from build123d import *

# Parameters (mm, degrees)
SKETCH1_R           = 2.25
BOSS_EXTRUDE1_DEPTH = 15
SKETCH2_R           = 2.25
CUT_EXTRUDE1_DEPTH  = 20
FILLET1_R           = 10


with BuildPart() as part:
    # Sketch1 → Boss-Extrude1 (new body)
    with BuildSketch(Plane(origin=(0, 0, 0), x_dir=(1, 0, 0), z_dir=(0, 1, 0))):
        with BuildLine():
            Line((-87.85411681, -7.5), (-62.85411681, -7.5))
            ThreePointArc((-62.85411681, -7.5), (1.256140371, -63.287535197), (63.102218661, -5))
            Line((63.102218661, -5), (73.102218661, -5))
            Line((73.102218661, -5), (73.102218661, -1))
            Line((73.102218661, -1), (55.290957669, -1))
            ThreePointArc((55.290957669, -1), (-55.3, 0), (55.290957669, 1))
            Line((55.290957669, 1), (73.102218661, 1))
            Line((73.102218661, 1), (73.102218661, 5))
            Line((73.102218661, 5), (63.102218661, 5))
            ThreePointArc((63.102218661, 5), (1.256140371, 63.287535197), (-62.85411681, 7.5))
            Line((-62.85411681, 7.5), (-87.85411681, 7.5))
            Line((-87.85411681, 7.5), (-87.85411681, -7.5))
        make_face()
        with Locations(Location((-80.85411681, 0, 0), (0, 0, 270))):
            Circle(SKETCH1_R, mode=Mode.SUBTRACT)
        with Locations(Location((-65.85411681, 0, 0), (0, 0, 270))):
            Circle(SKETCH1_R, mode=Mode.SUBTRACT)
    extrude(amount=BOSS_EXTRUDE1_DEPTH)

    # Sketch2 → Cut-Extrude1 (cut)
    with BuildSketch(Plane.XY.offset(5)):
        with Locations((68.102218661, 7.5)):
            Circle(SKETCH2_R)
    extrude(amount=-CUT_EXTRUDE1_DEPTH, mode=Mode.SUBTRACT)

    # Fillet1
    fillet1_edges = [part.edges().sort_by_distance(p)[0] for p in [
        (-62.85411681, 7.5, 7.5),
        (-62.85411681, 7.5, -7.5),
    ]]
    fillet(fillet1_edges, radius=FILLET1_R)


solid = part.part
CAD build for the part. Positions are in the model's coordinates, mm. A direction names the side the tool comes from. Give positions to 0.01 mm unless a question says otherwise; leave off trailing zeros. Loops run counter-clockwise (first coordinate to the right, second up) from the corner with the lowest first, then second, coordinate; pieces in that order, holes last. Notation, with made-up numbers: M 35,30.25 L 77,30.25 A25 ccw 77,65.25 Z; hole C -2,-9.5 d1. An arc over 180 degrees is marked long. Answer in a Markdown table with one row per item. Add a question column.
Item 1: Band-saw the part on C-C on z = 17.5. Give the cut face in (x, y), then the cut area to 3 significant figures.
Item 2: Tool access for faces 5 (the face through (64, 7, 1)), 6 (the face through (66, 9, 5)), 7 (the face through (-79, 7, -7.5)): list every direction of +Z, -Z, +X, -X, +Y, -Y with a clear straight run to the whole face (end or side of a thin tool).
Item 3: Drop flat-ended pins along their axis: P1, Ø10, axis at x = -23.5, z = -42.5, coming from the -Y side; P2, Ø1, axis at y = 6, z = 40.5, coming from the +X side; P3, Ø3, axis at x = 67.5, y = 8.5, coming from the -Z side; P4, Ø5, axis at x = 66.5, y = 9, coming from the +Z side. Give the stop position or say it passes through.
Item 4: Band-saw the part on A-A on x = 0. Give the cut face in (y, z).
Item 5: Probe probe 1 along X at (y, z) = (8.75, 0); probe 2 along Z at (x, y) = (1, 8.25); probe 3 along Z at (x, y) = (65, 10.5). List the from-to ranges inside material, lowest first.
Item 6: Mould opens along Y. For faces 1 (the face through (70, 9, -5)), 2 (the face through (-55.4, 0, -5)), 3 (the face through (65.854, 7.599, 3.028)), 4 (the face through (65.854, 7.599, -2.972)) say: +Y half, -Y half, draft (parallel to the pull), parting line (faces both ways), or undercut.
Item 7: Band-saw the part on D-D on x = -73. Give the cut face in (y, z).
Item 8: Band-saw the part on B-B on y = 7.5. Give the cut face in (x, z).
Reply:
| question | item | result |
|---|---|---|
| 1 | outline | M -60.83,0 L -52.46,0 L -52.46,15 L -60.83,15 Z; M 52.46,0 L 60.83,0 L 60.83,15 L 52.46,15 Z |
| 1 | area | 251 mm^2 |
| 2 | face 5 | +X, +Y, -Y |
| 2 | face 6 | +Z, +X, +Y, -Y |
| 2 | face 7 | -Z, -X, +Y, -Y |
| 3 | P1 | passes through |
| 3 | P2 | stops at x = 49.06 |
| 3 | P3 | stops at z = -5 |
| 3 | P4 | stops at z = 5 |
| 4 | outline | M 0,-63.3 L 15,-63.3 L 15,-55.3 L 0,-55.3 Z; M 0,55.3 L 15,55.3 L 15,63.3 L 0,63.3 Z |
| 5 | probe 1 | x = -87.85 to -83.1, -78.6 to -68.1, -63.6 to -55.3 |
| 5 | probe 2 | z = -63.29 to -55.29, 55.29 to 63.29 |
| 5 | probe 3 | z = -5 to -1, 1 to 5 |
| 6 | face 1 | draft |
| 6 | face 2 | -Y half |
| 6 | face 3 | undercut |
| 6 | face 4 | undercut |
| 7 | outline | M 0,-7.5 L 15,-7.5 L 15,7.5 L 0,7.5 Z |
| 8 | outline | M -87.85,-7.5 L -71.18,-7.5 A10 cw -61.47,-15.11 A63.3 ccw 63.1,-5 L 65.85,-5 L 65.85,-1 L 55.29,-1 A55.3 cw long 55.29,1 L 65.85,1 L 65.85,5 L 63.1,5 A63.3 ccw -61.47,15.11 A10 cw -71.18,7.5 L -87.85,7.5 Z; M 70.35,-5 L 73.1,-5 L 73.1,-1 L 70.35,-1 Z; M 70.35,1 L 73.1,1 L 73.1,5 L 70.35,5 Z; hole C -80.85,0 d4.5; hole C -65.85,0 d4.5 |
